Work out the finished part from the listing and answer in its coordinate system (mm). A direction names the side the tool comes from. Coordinates: 2 decimals unless noted, no trailing zeros. Loops run counter-clockwise (first coordinate to the right, second up) from the corner with the lowest first, then second, coordinate; pieces in that order, holes last. Notation, with made-up numbers: (14.25, 40.25) - (48.25, 40.25) arc R14 ccw to (48.25, 48.25) - close; hole circle Ø7 at (88, 31). An arc over 180 degrees is marked (long way). Write each question's results on one line, items separated by ' | '. Start each with the question number.
1. A cutting plane is placed at A-A on x = -12. Determine the outline of the cut face in (y, z), then the cut area to 3 significant figures.
2. Determine the mould class of faces 1 (the conical face through (-10.28, -177.46, -66.46)), 2 (the flat face through (-10.9, -145, 69)), 3 (the cylindrical face through (-13.956, -130.975, 56.686)) for opening direction Y: released by +Y, released by -Y, zero draft, split by the parting line, or undercut.
3. Find the intervals of material crossed by line 1 along Z through (x, y) = (-16, -129.9); line 2 along Z through (x, y) = (-13, -170.9); line 3 along Y through (x, z) = (-14.25, 53.5), in increasing order. Write a range as [from, to].
4. A cutting plane is placed at D-D on z = 23. Determine the outline of the cut face in (x, y).
5. Each of these flat-tipped pins is pushed along its axis until it touches: P1, Ø3.5, axis at y = -129.9, z = 55, coming from the -X side; P2, Ø6, axis at x = -10.5, z = 22.5, coming from the -Y side. Where does it stop, or does it pass through?
6. A cutting plane is placed at B-B on y = -129.9. Determine the outline of the cut face in (x, z).
7. Which of the six approach directions +Z, -Z, +X, -X, +Y, -Y give full straight-line access (tool end or side, diameter ignored) to faces 4 (the flat face through (-9.9, -171, 55)), 5 (the conical face through (-10.28, -113.44, -66.56))?
8. A cutting plane is placed at C-C on z = -50. Determine the outline of the cut face in (x, y).
from build123d import *

# Parameters (mm, degrees)
SKETCH156_W             = 75
SKETCH156_H             = 144
PAD044_DEPTH            = 10
FILLET024_R             = 10
CHAMFER009_SIZE         = 6
SKETCH164_R             = 2
POCKET055_DEPTH         = 8
BODY015_PLACEMENT_ANGLE = 180


with BuildPart() as part:
    # Sketch156 → Pad044 (new body)
    with BuildSketch(Plane.YZ):
        with Locations((0.5, 0)):
            Rectangle(SKETCH156_W, SKETCH156_H)
    extrude(amount=PAD044_DEPTH)

    # Fillet024
    fillet024_edges = [part.edges().sort_by_distance(p)[0] for p in [
        (5, 38, -72),
        (5, -37, -72),
        (5, -37, 72),
        (5, 38, 72),
    ]]
    fillet(fillet024_edges, radius=FILLET024_R)

    # Chamfer009
    chamfer009_edges = [part.edges().sort_by_distance(p)[0] for p in [
        (0, 0.5, 72),
        (0, -37, 0),
        (0, 38, 0),
        (0, 0.5, -72),
    ]]
    chamfer(chamfer009_edges, length=CHAMFER009_SIZE)

    # Sketch164 (on Face4 of Chamfer009) → Pocket055 (cut)
    with BuildSketch(Plane.YZ.offset(10)):
        with Locations((-15, 55)):
            Circle(SKETCH164_R)
        with Locations((26, 55)):
            Circle(SKETCH164_R)
        with Locations((-15, -50)):
            Circle(SKETCH164_R)
        with Locations((26, -50)):
            Circle(SKETCH164_R)
    extrude(amount=-POCKET055_DEPTH, mode=Mode.SUBTRACT)


with BuildPart() as part_1:
    # Body015 placement: moved
    add(part.part.moved(Location((-7.9, -144.9, 0))).rotate(Axis((-7.9, -144.9, 0), (0, 0, 1)), BODY015_PLACEMENT_ANGLE))


solid = part_1.part
Values:
1) outline: (-181, -62) arc R8.1 ccw to (-172.9, -70.1) - (-117.9, -70.1) arc R8.1 ccw to (-109.8, -62) - (-109.8, 62) arc R8.1 ccw to (-117.9, 70.1) - (-172.9, 70.1) arc R8.1 ccw to (-181, 62) - close; hole circle Ø4 at (-170.9, -50); hole circle Ø4 at (-170.9, 55); hole circle Ø4 at (-129.9, -50); hole circle Ø4 at (-129.9, 55) | area: 9,880 mm^2
2) face 1: released by -Y | face 2: zero draft | face 3: undercut
3) line 1: [-72, -52], [-48, 53], [57, 72] | line 2: [-71.1, -52], [-48, 53], [57, 71.1] | line 3: [-182.9, -172.22], [-169.58, -131.22], [-128.58, -107.9]
4) outline: (-17.9, -182.9) - (-13.9, -182.9) - (-7.9, -176.9) - (-7.9, -113.9) - (-13.9, -107.9) - (-17.9, -107.9) - close
5) P1: x = -9.9 | P2: y = -182.5
6) outline: (-17.9, -72) - (-13.9, -72) - (-7.9, -66) - (-7.9, 66) - (-13.9, 72) - (-17.9, 72) - (-17.9, 57) - (-9.9, 57) - (-9.9, 53) - (-17.9, 53) - (-17.9, -48) - (-9.9, -48) - (-9.9, -52) - (-17.9, -52) - close
7) face 4: -X | face 5: -Z, +X, +Y
8) outline: (-17.9, -182.9) - (-13.9, -182.9) - (-7.9, -176.9) - (-7.9, -113.9) - (-13.9, -107.9) - (-17.9, -107.9) - (-17.9, -127.9) - (-9.9, -127.9) - (-9.9, -131.9) - (-17.9, -131.9) - (-17.9, -168.9) - (-9.9, -168.9) - (-9.9, -172.9) - (-17.9, -172.9) - close
